```python
from build123d import *

# Parameters (mm, degrees)
F0_R      = 127
F1_DEPTH  = 381
F2_R      = 15.24
F3_W      = 126.0042116046
F3_H      = 33.7627371773
F4_DEPTH  = 63.5
F5_W      = 126.0042116046
F5_H      = 63.5
F6_DEPTH  = 127
F7_W      = 126.0042116046
F7_H      = 27.3971298127
F8_DEPTH  = 355.6
F9_DEPTH  = 25.4
F11_DEPTH = 127
F12_W     = 27.3971298127
F12_H     = 419.1
F13_DEPTH = 127
F14_R     = 17.4895868551
F14_R_2   = 27.5583251685
F15_DEPTH = 50.8


with BuildPart() as f1:
    # F0 (on Top) → F1 (new body)
    with BuildSketch(Plane.XY):
        with Locations((-18.0272441357, 8.4358751774)):
            Circle(F0_R)
    extrude(amount=F1_DEPTH)

    # F2
    f2_edges = [f1.edges().sort_by_distance(p)[0] for p in [
        (-145.027244, 8.435875, 381),
    ]]
    fillet(f2_edges, radius=F2_R)

    # F3 (on face) → F4 (join)
    with BuildSketch(Plane.XY.offset(381)):
        with Locations((-20.0667567551, 3.8541001268)):
            Rectangle(F3_W, F3_H)
    extrude(amount=F4_DEPTH)

    # F5 (on face) → F6 (join)
    with BuildSketch(Plane.XZ.offset(13.0272684619)):
        with Locations((-20.0667567551, 412.75)):
            Rectangle(F5_W, F5_H)
    extrude(amount=F6_DEPTH)

    # F7 (on face) → F8 (join)
    with BuildSketch(Plane(origin=(0, 0, 381), x_dir=(1, 0, 0), z_dir=(0, 0, -1))):
        with Locations((-20.0667567551, 126.3287035555)):
            Rectangle(F7_W, F7_H)
    extrude(amount=F8_DEPTH)

    # F9 (add): a face of the model
    f9_faces = [f1.faces().sort_by_distance(p)[0] for p in [
        (-83.0688625574, -135.5385106419, 234.95),
    ]]
    extrude(f9_faces, amount=F9_DEPTH)

    # F10 (on face) → F11 (join)
    with BuildSketch(Plane(origin=(-108.4688625574, 0, 0), x_dir=(0, -1, 0), z_dir=(-1, 0, 0))):
        Polygon((140.0272684619, 25.4), (140.0272684619, 444.5), (112.6301386492, 444.5), (112.6301386492, 381), (112.6301386492, 25.4), align=None)
    extrude(amount=F11_DEPTH)

    # F12 (on face) → F13 (join)
    with BuildSketch(Plane.YZ.offset(42.9353490472)):
        with Locations((-126.3287035555, 234.95)):
            Rectangle(F12_W, F12_H)
    extrude(amount=F13_DEPTH)

    # F14 (on face) → F15 (cut)
    with BuildSketch(Plane.XZ.offset(140.0272684619)):
        with Locations((-167.4611866474, 399.9962210655)):
            Circle(F14_R)
        with Locations((97.0467850566, 406.0656428337)):
            Circle(F14_R_2)
        with BuildLine():
            add(Edge.make_bspline(
                [(-176.0322153568, 189.0380978584), (-201.9253380349, 151.3628030109), (-24.8268478885, 23.085444119), (238.6265275345, 243.979797102), (-143.4799308709, 236.4026792268), (-176.0322153568, 189.0380978584)],
                knots=[0, 0, 0, 0, 0.3093685357, 0.6110684405, 1, 1, 1, 1], degree=3))
        make_face()
    extrude(amount=-F15_DEPTH, mode=Mode.SUBTRACT)


solid = f1.part
```
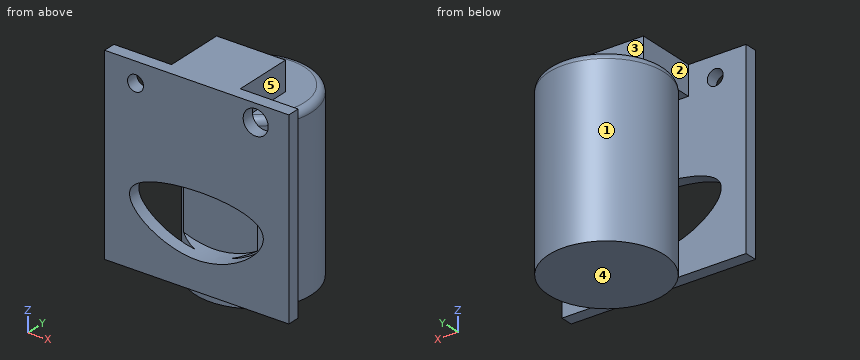
Here's how the part is built. I have some questions about the finished solid (model axes, mm). Face numbers are marked on the shaded views. A direction names the side the tool comes from. Coordinates: 2 decimals unless noted, no trailing zeros. Order: outer loops, then holes, each group sorted by start corner. A loop starts at its lowest first (then second) coordinate and runs counter-clockwise, first axis right, second up. Notation, with made-up numbers: M 7.25,-39.5 L 13.25,-39.5 A25 cw 13.25,-14.5 Z; hole C -37,5 d6. An arc over 180 degrees is marked long. Answer as a JSON object with one key per item and string values. Group by question number.
(1) If we mould it in two halves opening along Y, with no side actions, what happens to the marked faces 1, 2 and 3? For each: released by +Y, released by -Y, zero draft, split by the parting line, or undercut.
(2) I need wall thicknesses on probe 1 along Z at (x, y) = (77, -114.5); probe 2 along X at (y, z) = (3, 34.5); probe 3 along X at (y, z) = (-96.5, 413.5). Which ranges of each line are inside material? Lowest first, please.
(3) Suppose I cut it at B-B, the plane x = 144. Please give me the cut outline in (y, z).
(4) For pin 1 (4 mm diameter, centred on y = -72.5, z = 271.5, fed in from +X); pin 2 (12 mm diameter, centred on x = 97, z = 189.5, fed in from +Y); pin 3 (19 mm diameter, centred on x = -70.5, z = 413.5, fed in from +Y), each with a flat end and sliding along its axis, tell me the tip position at first contact or that it passes through.
(5) Suppose I cut it at A-A, the plane z = 195.5. State how many separate pieces and enclosed holes the cut face has, then the cut area to 3 significant figures.
(6) Suppose I cut it at C-C, the plane z = 348. Please give me the cut outline in (x, y).
(7) Which directions (+Z, -Z, +X, -X, +Y, -Y) give clear straight access to the entire face, cutting with the end or side of a thin tool? Please do the marked faces 4 and 5.
Values found:
{
 "1": {"face 1": "undercut", "face 2": "zero draft", "face 3": "released by +Y"},
 "2": {"probe 1": "z = 25.4 to 124.76, 213.08 to 387.16, 424.98 to 444.5", "probe 2": "x = -144.91 to 108.86", "probe 3": "x = -108.47 to 42.94"},
 "3": {"outline": "M -140.03,25.4 L -112.63,25.4 L -112.63,444.5 L -140.03,444.5 Z"},
 "4": {"pin 1": "stops at x = 81.46", "pin 2": "stops at y = 73.57", "pin 3": "stops at y = 20.74"},
 "5": {"separate pieces": "3", "enclosed holes": "0", "area": "50,900 mm^2"},
 "6": {"outline": "M -235.47,-140.03 L 169.94,-140.03 L 169.94,-112.63 L 20.34,-112.63 A127 ccw long -56.39,-112.63 L -235.47,-112.63 Z"},
 "7": {"face 4": "-Z, +X, -X, +Y, -Y", "face 5": "+Z, +X, +Y"}
}
